Geometry check sheet. Reference: drawing and pictorial views, mm from the part's lowest x, y, z. A direction names the side the tool comes from. Give positions to 0.01 mm unless a question says otherwise; leave off trailing zeros. Write each loop counter-clockwise with the first axis right and the second up, starting at its lowest first coordinate (ties: lowest second). Pieces come first, ordered by that corner, then holes. Notation, with made-up numbers: (19, 65) -> (42, 65) arc R9 ccw to (42, 74) -> close; hole circle Ø2 at (-26, -18.75). An arc over 180 degrees is marked (long way). Return JSON: item names as keys, results as strings.
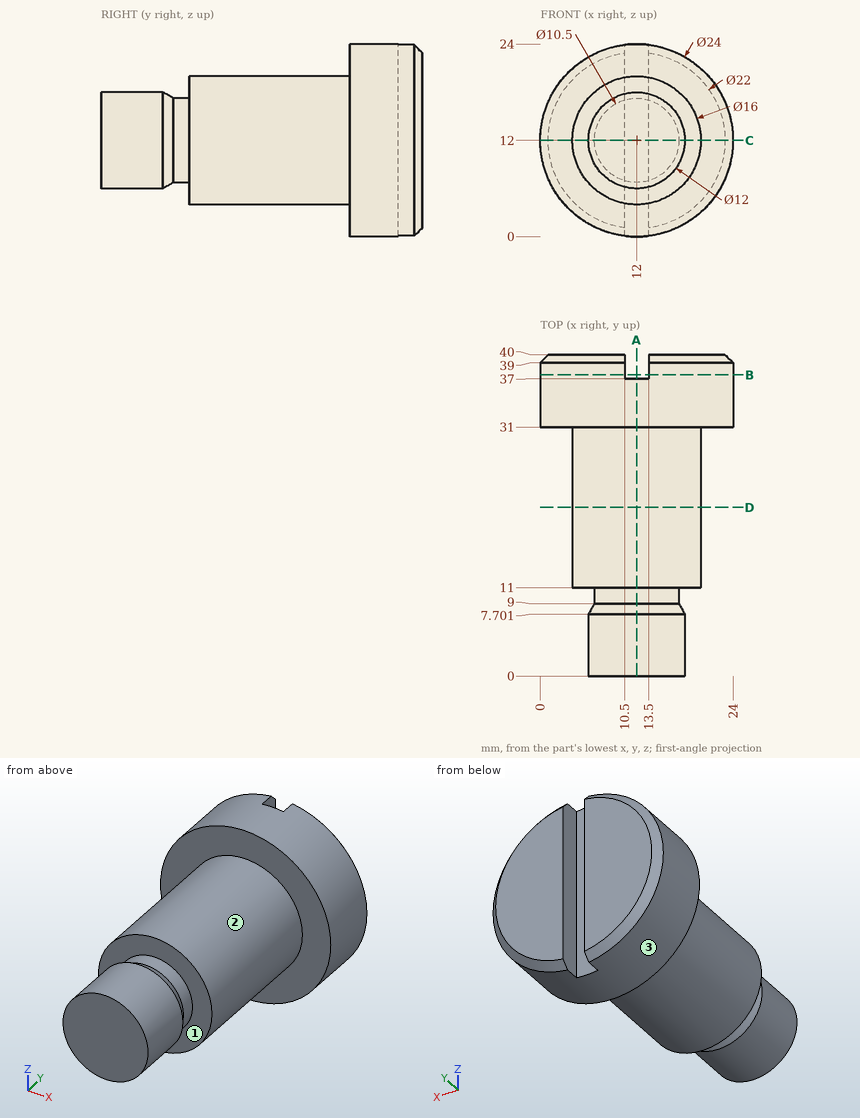
(1) Cross-section at C-C on z = 12. Enter the section's corners in (x, y), then the cut area to 3 significant figures.
Reply:
{"outline": "(0, 31) -> (4, 31) -> (4, 11) -> (6.75, 11) -> (6.75, 9) -> (6, 7.7) -> (6, 0) -> (18, 0) -> (18, 7.7) -> (17.25, 9) -> (17.25, 11) -> (20, 11) -> (20, 31) -> (24, 31) -> (24, 39) -> (23, 40) -> (13.5, 40) -> (13.5, 37) -> (10.5, 37) -> (10.5, 40) -> (1, 40) -> (0, 39) -> close", "area": "654 mm^2"}
(2) Thickness scan on L1, parallel to Y at x = 17, z = 19.5; L2, parallel to Y at x = 7.25, z = 16.75; L3, parallel to Z at x = 11.5, y = 35.5. Record the ranges inside material, lowest first.
Reply:
{"L1": "31 to 40", "L2": "11 to 40", "L3": "0.01 to 23.99"}
(3) Cross-section at B-B on y = 37.5. Enter the section's corners in (x, z), then the cut area to 3 significant figures.
Reply:
{"outline": "(10.5, 0.09) -> (10.5, 23.91) arc R12 ccw to start; (13.5, 0.09) arc R12 ccw to (13.5, 23.91) -> close", "area": "381 mm^2"}
(4) Cross-section at A-A on x = 12. Enter the section's corners in (y, z), then the cut area to 3 significant figures.
Reply:
{"outline": "(0, 6) -> (7.7, 6) -> (9, 6.75) -> (11, 6.75) -> (11, 4) -> (31, 4) -> (31, 0) -> (37, 0) -> (37, 24) -> (31, 24) -> (31, 20) -> (11, 20) -> (11, 17.25) -> (9, 17.25) -> (7.7, 18) -> (0, 18) -> close", "area": "592 mm^2"}
(5) Set-up check for the marked faces 1, 2 and 3: record each of +Z, -Z, +X, -X, +Y, -Y from which the full face is reachable in a straight line by a thin tool's end or side.
Reply:
{"face 1": "none", "face 2": "-Y", "face 3": "+Y, -Y"}
(6) Cross-section at D-D on y = 21. Enter the section's corners in (x, z).
Reply:
{"outline": "circle Ø16 at (12, 12)"}
(7) Depth check by flat-ended pin: pin 1 Ø8 at (x, y) = (14, 10.5) entering from +Z; pin 2 Ø12 at (y, z) = (30.5, 13.5) entering from -X; pin 3 Ø3 at (y, z) = (15.5, 19.5) entering from +X; pin 4 Ø1.5 at (x, z) = (5, 12) entering from -Y. Enter the tip coordinate at first touch or a pass-through.
Reply:
{"pin 1": "z = 20", "pin 2": "x = 0", "pin 3": "x = 17.29", "pin 4": "y = 11"}
